Source: three-view drawing plus pictorial views. Frame: mm from the lowest corner of the part. Give positions to 0.01 mm unless a question says otherwise; leave off trailing zeros. Order: outer loops, then holes, each group sorted by start corner. A loop starts at its lowest first (then second) coordinate and runs counter-clockwise, first axis right, second up. Notation, with made-up numbers: (22, -18) -> (67, -18) arc R18 cw to (67, -12) -> close; hole circle Ø11 at (31.25, -36). An arc over 180 degrees is marked (long way). One line per question, with ' | ' between items.
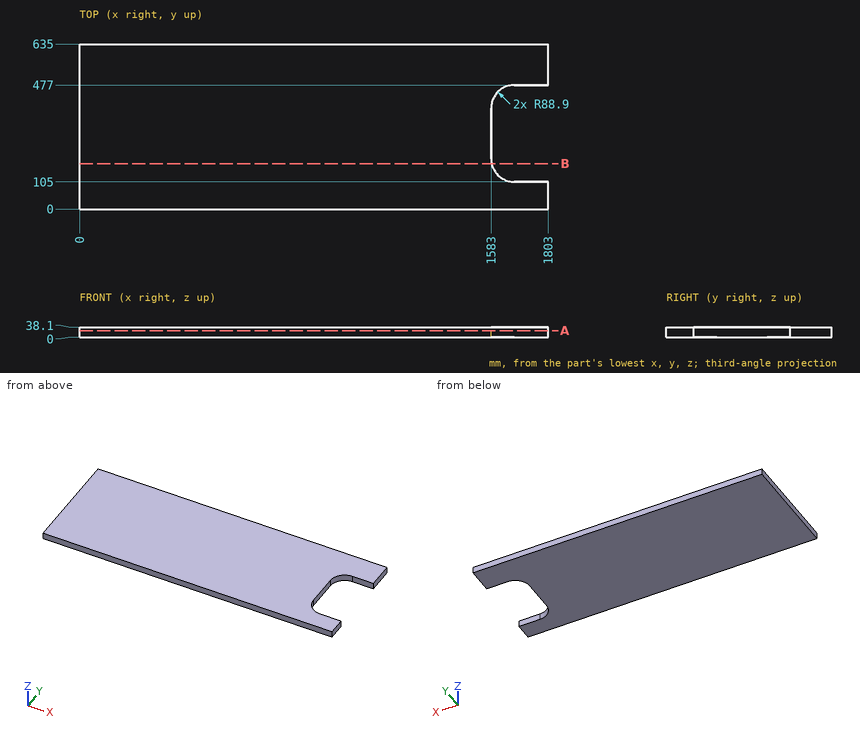
1) Section A-A on z = 24.5. Return loops of the section in (x, y).
Check result:
outline: (0, 0) -> (1803, 0) -> (1803, 105) -> (1671.9, 105) arc R88.9 cw to (1583, 193.9) -> (1583, 388.1) arc R88.9 cw to (1671.9, 477) -> (1803, 477) -> (1803, 635) -> (0, 635) -> close
2) Contact query for a flat-ended pin moving along its axis: pin 1 Ø1 at (y, z) = (196.5, 22) entering from +X. Output: stop coordinate, or through.
Check result:
pin 1: stops at x = 1583
3) Section B-B on y = 175. Return loops of the section in (x, z).
Check result:
outline: (0, 0) -> (1585.03, 0) -> (1585.03, 38.1) -> (0, 38.1) -> close
4) Material intervals for probe 1 along Y at (x, z) = (1684, 15.5); probe 2 along X at (y, z) = (352.5, 28); probe 3 along Y at (x, z) = (1663, 22), sorted ascending. Write a range as from..to.
Check result:
probe 1: y = 0..105, 477..635 | probe 2: x = 0..1583 | probe 3: y = 0..105.45, 476.55..635
